Verification items for the finished model (mm, model axes). A direction names the side the tool comes from. Give positions to 0.01 mm unless a question says otherwise; leave off trailing zeros. Loops run counter-clockwise (first coordinate to the right, second up) from the corner with the lowest first, then second, coordinate; pieces in that order, holes last. Notation, with made-up numbers: M -22.75,-15 L 16.25,-15 A11 ccw 16.25,-6 Z; hole C 43,31.25 d2. An arc over 180 degrees is marked long. Answer in a Markdown table with one row per item.
Autodesk Inventor part; units mm, degrees
ref_plane "YZ Plane" through (0, 0, 0) normal (1, 0, 0) x (0, 1, 0)
ref_plane "XZ Plane" through (0, 0, 0) normal (0, 1, 0) x (-1, 0, 0)
ref_plane "XY Plane" through (0, 0, 0) normal (0, 0, 1) x (1, 0, 0)
sketch "Sketch1" plane through (0, 0, 0) normal (0, 1, 0) x (-1, 0, 0)
  line L0 (0, 0) -> (-25.4, 0)
  line L1 (-25.4, 0) -> (-25.4, 76.2)
  line L2 (-25.4, 76.2) -> (0, 76.2)
  line L3 (0, 76.2) -> (0, 0)
  line L4 (-25.4, 76.2) -> (-50.8, 76.2)
  line L5 (-50.8, 76.2) -> (-50.8, 50.8)
  line L6 (-50.8, 50.8) -> (-25.4, 50.8)
  line L7 (-25.4, 50.8) -> (-25.4, 76.2)
  circle A0 centre (-12.7, 12.7) radius 5.2917
  circle A1 centre (-38.1, 63.5) radius 5.2917
  circle A2 centre (-12.7, 38.1) radius 5.2917
  circle A3 centre (-12.7, 63.5) radius 5.2917
  dimension "d0" = 76.2
  dimension "d1" = 25.4
  dimension "d2" = 25.4
  dimension "d3" = 25.4
  dimension "d5" = 38.1
  dimension "d7" = 25.4
  dimension "d8" = 25.4
  dimension "d11" = 12.7
  dimension "d12" = 12.7
  dimension "d13" = 12.7
  dimension "d14" = 10.5833
  dimension "d15" = 10.5833
  dimension "d16" = 10.5833
  dimension "d17" = 10.5833
  dimension "d18" = 12.7
  dimension "d19" = 25.4
  dimension "d20" = 12.7
extrude "Extrusion1" add sketch "Sketch1" along normal blind 2.54
equation "\"d15\" = d14"
equation "\"d16\" = d14"
equation "\"d17\" = d14"
properties part number "bracing 2x3"
Item 1: Sectioned sample at D-D (z = 38.1). Record the cut outline in (x, y).
Reported:
| item | result |
|---|---|
| outline | M 0,0 L 7.41,0 L 7.41,2.54 L 0,2.54 Z; M 17.99,0 L 25.4,0 L 25.4,2.54 L 17.99,2.54 Z |
Item 2: Scan lines: L1, parallel to Z at x = 12.7, y = 0.65; L2, parallel to Z at x = 8, y = 1.15; L3, parallel to X at y = 1.4, z = 60. Record each from-to range of solid material in increasing order. Write a range as [from, to].
Reported:
| item | result |
|---|---|
| L1 | z = [0, 7.41], [17.99, 32.81], [43.39, 58.21], [68.79, 76.2] |
| L2 | z = [0, 10.27], [15.13, 35.67], [40.53, 61.07], [65.93, 76.2] |
| L3 | x = [0, 8.73], [16.67, 34.13], [42.07, 50.8] |
Item 3: Go/stop test with a flat-tipped pin: pin 1 (9.5 mm diameter, centred on x = 38.1, z = 63.5, fed in from +Y). Record where the tip stops, or that it passes through.
Reported:
| item | result |
|---|---|
| pin 1 | passes through |
Item 4: Release check for a two-part mould opening along Z. For faces 1 (the cylindrical face through (13.389, 1.252, 7.453)), 2 (the flat face through (20, 2.54, 47)), 3 (the flat face through (38, 1, 50.8)) record: released by +Z, released by -Z, zero draft, split by the parting line, or undercut.
Reported:
| item | result |
|---|---|
| face 1 | undercut |
| face 2 | zero draft |
| face 3 | released by -Z |
Item 5: Sectioned sample at B-B (y = 1.85). Record the cut outline in (x, z), and give its area (3 significant figures).
Reported:
| item | result |
|---|---|
| outline | M 0,0 L 25.4,0 L 25.4,50.8 L 50.8,50.8 L 50.8,76.2 L 0,76.2 Z; hole C 12.7,12.7 d10.58; hole C 12.7,38.1 d10.58; hole C 12.7,63.5 d10.58; hole C 38.1,63.5 d10.58 |
| area | 2,230 mm^2 |
Item 6: Sectioned sample at A-A (z = 63.5). Record the cut outline in (x, y), and give its area (3 significant figures).
Reported:
| item | result |
|---|---|
| outline | M 0,0 L 7.41,0 L 7.41,2.54 L 0,2.54 Z; M 17.99,0 L 32.81,0 L 32.81,2.54 L 17.99,2.54 Z; M 43.39,0 L 50.8,0 L 50.8,2.54 L 43.39,2.54 Z |
| area | 75.3 mm^2 |
Item 7: Tool access check on faces 4 (the cylindrical face through (13.847, 1.252, 68.666)), 5 (the flat face through (25.4, 1, 25)). Record the directions out of +Z, -Z, +X, -X, +Y, -Y that give a thin tool (end or side, any length) a straight path to the whole face; none if there is none.
Reported:
| item | result |
|---|---|
| face 4 | +Y, -Y |
| face 5 | -Z, +X, +Y, -Y |
Item 8: Sectioned sample at C-C (x = 38.1). Record the cut outline in (y, z), and give its area (3 significant figures).
Reported:
| item | result |
|---|---|
| outline | M 0,50.8 L 2.54,50.8 L 2.54,58.21 L 0,58.21 Z; M 0,68.79 L 2.54,68.79 L 2.54,76.2 L 0,76.2 Z |
| area | 37.6 mm^2 |
